Autodesk Inventor part; units mm, degrees
ref_plane "YZ Plane" through (0, 0, 0) normal (1, 0, 0) x (0, 1, 0)
ref_plane "XZ Plane" through (0, 0, 0) normal (0, 1, 0) x (-1, 0, 0)
ref_plane "XY Plane" through (0, 0, 0) normal (0, 0, 1) x (1, 0, 0)
sketch "Boceto1" plane through (0, 0, 0) normal (0, 1, 0) x (-1, 0, 0)
  line L0 (100, 100) -> (-100, 100)
  line L1 (-100, 100) -> (-100, -100)
  line L2 (-100, -100) -> (100, -100)
  line L3 (100, -100) -> (100, 100)
  line L4 (100, 100) -> (-100, -100) construction
  line L5 (-100, 100) -> (100, -100) construction
  point P0 (0, 0)
  dimension "d0" = 200
  dimension "d1" = 200
extrude "Extrusión1" add sketch "Boceto1" along normal blind 20
sketch "Boceto2" plane through (0, 20, 0) normal (0, 1, 0) x (1, 0, 0)
  circle A0 centre (-11.5239, -30.0616) radius 3
  circle A1 centre (11.4761, -30.0616) radius 3
  circle A2 centre (-11.5239, -60.0616) radius 3
  circle A3 centre (11.4761, -60.0616) radius 3
  line L0 (-0.0239, -45.0616) -> (-35.0239, -45.0616)
  line L1 (-35.0239, -45.0616) -> (-35.0239, -80.0616)
  line L2 (-0.0239, -45.0616) -> (34.9761, -45.0616)
  line L3 (-11.5239, -30.0616) -> (11.4761, -60.0616)
  line L4 (-11.5239, -60.0616) -> (11.4761, -30.0616)
  line L5 (34.9761, -20.0616) -> (-35.0239, -20.0616)
  line L6 (-35.0239, -20.0616) -> (-35.0239, -80.0616)
  line L7 (34.9761, -80.0616) -> (34.9761, -20.0616)
  line L8 (-105, -100.0616) -> (105, -100.0616)
  line L9 (-105.0239, -80.0616) -> (104.9761, -80.0616)
  line L10 (-35.0239, -80.0616) -> (34.9761, -80.0616)
  line L11 (105, -100.0616) -> (95.8154, -100.0616)
  line L12 (-105.0239, -80.0616) -> (104.9761, -80.0616)
  line L13 (105, -80.0616) -> (-105, -80.0616)
  line L14 (-105, -100.0616) -> (105, -100.0616)
  line L15 (105, -90.0616) -> (94.0798, -90.0616)
  line L16 (-105, -100.0616) -> (105, -100.0616)
  line L17 (-105, -80.0616) -> (105, -80.0616)
  line L18 (105, -80.0616) -> (105, -100.0616)
  line L19 (105, -100.0616) -> (-105, -100.0616)
  line L20 (-105, -100.0616) -> (-105, -80.0616)
  line L21 (-100, 100) -> (-100, -100)
  line L22 (-100, -100) -> (100.4077, -100)
  point P0 (0, 0)
  point P1 (0, -10.0616)
  point P2 (0, -90.0616)
  point P3 (-0.0478, -80.0616)
  dimension "d4" = 20
  dimension "d5" = 20
  dimension "d6" = 30
  dimension "d7" = 30
  dimension "d8" = 20
  dimension "d9" = 35
  dimension "d10" = 35
  dimension "d11" = 60
extrude "Extrusión2" cut sketch "Boceto2" against normal blind 10
sketch "Boceto3" plane through (0, 20, 0) normal (0, 1, 0) x (1, 0, 0)
  circle A0 centre (-11.5239, -30.0616) radius 3
  circle A1 centre (-11.5239, -30.0616) radius 3
  circle A2 centre (11.4761, -30.0616) radius 3
  circle A3 centre (11.4761, -30.0616) radius 3
  circle A4 centre (11.4761, -60.0616) radius 3
  circle A5 centre (11.4761, -60.0616) radius 3
  circle A6 centre (-11.5239, -60.0616) radius 3
  point P0 (0, 0)
extrude "Extrusión3" cut sketch "Boceto3" against normal blind 20
sketch "Boceto4" plane through (0, 20, 0) normal (0, 1, 0) x (1, 0, 0)
  circle A0 centre (-51.75, 78.25) radius 1.75
  line L0 (-50, 70) -> (-60, 70)
  line L1 (-60, 70) -> (-60, 80)
  line L2 (-60, 80) -> (-50, 80)
  line L3 (-50, 80) -> (-50, 70)
  line L4 (-50, 70) -> (-60, 80) construction
  line L5 (-60, 70) -> (-50, 80) construction
  line L6 (-105, 90) -> (-105, -90)
  circle A1 centre (-58.25, 71.75) radius 1.75
  line L7 (0, 90) -> (0, 77.3124)
  circle A2 centre (51.75, 78.25) radius 1.75
  line L8 (50, 70) -> (60, 70)
  line L9 (60, 70) -> (60, 80)
  line L10 (60, 80) -> (50, 80)
  line L11 (50, 80) -> (50, 70)
  line L12 (50, 70) -> (60, 80) construction
  line L13 (60, 70) -> (50, 80) construction
  circle A3 centre (58.25, 71.75) radius 1.75
  line L14 (100, 100) -> (-100, 100)
  line L15 (-100, 100) -> (-100, -80.0616)
  line L16 (100, -80.0616) -> (100, 100)
  point P0 (0, 0)
  point P1 (0, 0)
  point P2 (-60, 75)
  point P3 (60, 75)
  dimension "d16" = 3.5
  dimension "d18" = 1.75
  dimension "d19" = 1.75
  dimension "d20" = 1.75
  dimension "d21" = 1.75
  dimension "d22" = 10
  dimension "d23" = 10
  dimension "d25" = 20
  dimension "d26" = 40
  dimension "d27" = 40
hole "Agujero1" at (-58.25, 20, -71.75) at (-51.75, 20, -78.25) at (58.25, 20, -71.75) at (51.75, 20, -78.25) direction (0, -1, 0) diameter 3.5 end through all
sketch "Boceto5" plane through (0, 20, 0) normal (0, 1, 0) x (1, 0, 0)
  line L0 (0, 90) -> (0, 68.25)
  circle A0 centre (-51.75, 78.25) radius 1.75
  line L1 (-50, 78.25) -> (-50, 100)
  circle A1 centre (-58.25, 71.75) radius 1.75
  line L2 (-60, 71.75) -> (-60, 100)
  line L3 (-60, 100) -> (-70, 100)
  line L4 (-50, 100) -> (-40, 100)
  line L5 (-40, 100) -> (-40, 60)
  line L6 (-40, 60) -> (-70, 60)
  line L7 (-70, 60) -> (-70, 100)
  line L8 (-70, 100) -> (-40, 100)
  circle A2 centre (51.75, 78.25) radius 1.75
  line L9 (50, 78.25) -> (50, 100)
  circle A3 centre (58.25, 71.75) radius 1.75
  line L10 (60, 71.75) -> (60, 100)
  line L11 (60, 100) -> (70, 100)
  line L12 (50, 100) -> (40, 100)
  line L13 (40, 100) -> (40, 60)
  line L14 (40, 60) -> (70, 60)
  line L15 (70, 60) -> (70, 100)
  line L16 (70, 100) -> (40, 100)
  point P0 (0, 0)
  dimension "d38" = 10
  dimension "d39" = 10
  dimension "d40" = 40
extrude "Extrusión4" cut sketch "Boceto5" against normal blind 10
ref_plane "Plano de trabajo1" through (0, 0, -100) normal (-1, 0, 0) x (0, 0, 1)
ref_plane "Plano de trabajo2" through (100, 0, 0) normal (0, 0, -1) x (-1, 0, 0)
sketch "Boceto7" plane through (0, 0, 0) normal (0, -1, 0) x (1, 0, 0)
  circle A0 centre (10, -10) radius 1.75
  line L0 (6.803, 0) -> (14.6069, 0)
  line L1 (0, 0) -> (0, -4.8284)
  line L2 (0, 0) -> (20.0354, 0)
  circle A1 centre (10, 10) radius 1.75
  line L3 (0, 0) -> (0, 4.8284)
  circle A2 centre (-10, -10) radius 1.75
  circle A3 centre (-10, 10) radius 1.75
  dimension "d52" = 3.5
  dimension "d54" = 10
  dimension "d55" = 10
hole "Agujero2" at (10, 0, -10) at (10, 0, 10) at (-10, 0, 10) at (-10, 0, -10) direction (0, 1, 0) diameter 3.5 end through all
sketch "Boceto8" plane through (0, 0, 0) normal (0, -1, 0) x (1, 0, 0)
  line L0 (-15, 15) -> (15, 15)
  line L1 (15, 15) -> (15, -15)
  line L2 (15, -15) -> (-15, -15)
  line L3 (-15, -15) -> (-15, 15)
  line L4 (-15, 15) -> (15, -15) construction
  line L5 (15, 15) -> (-15, -15) construction
  point P0 (0, 0)
  dimension "d63" = 30
  dimension "d64" = 30
extrude "Extrusión5" cut sketch "Boceto8" against normal blind 10
sketch "Boceto9" plane through (0, 0, 0) normal (0, -1, 0) x (1, 0, 0)
  circle A0 centre (85, -10) radius 1.75
  line L0 (100, 100) -> (100, -100)
  line L1 (140, 0) -> (-140, 0)
  circle A1 centre (85, 10) radius 1.75
  line L2 (0, 0) -> (0, 9.4908)
  circle A2 centre (-85, -10) radius 1.75
  circle A3 centre (-85, 10) radius 1.75
  line L3 (0, 0) -> (6.3157, 6.3157)
  line L4 (0, 0) -> (8.9318, 0) construction
  circle A4 centre (10, 85) radius 1.75
  circle A5 centre (-10, -85) radius 1.75
  line L5 (0, 0) -> (5.9531, -5.9531)
  line L6 (0, 0) -> (8.419, 0) construction
  circle A6 centre (10, -85) radius 1.75
  circle A7 centre (-10, 85) radius 1.75
  dimension "d67" = 3.5
  dimension "d68" = 15
  dimension "d69" = 10
  dimension "d70" = 45
  dimension "d71" = 45
hole "Agujero3" at (-10, 0, 85) at (10, 0, 85) at (85, 0, 10) at (85, 0, -10) at (-85, 0, 10) at (-85, 0, -10) at (-10, 0, -85) at (10, 0, -85) direction (0, 1, 0) diameter 3.5 end through all
split "Dividir3" plane through (100, 0, 0) removes the side toward (0, 0, -1)
split "Dividir4" plane through (0, 0, -100) removes the side toward (1, 0, 0)
properties part number "base_front_3"
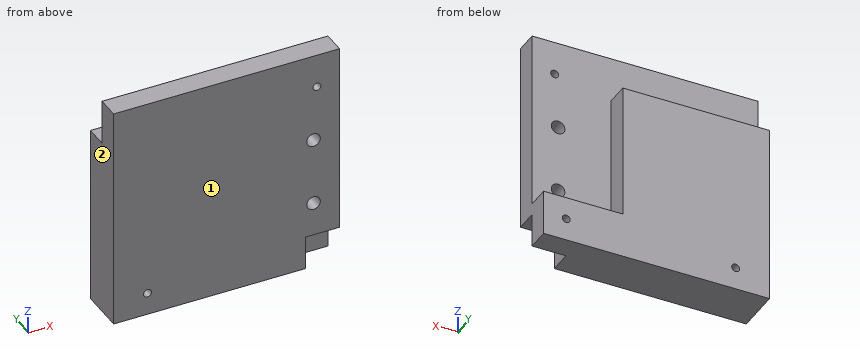
CAD build for the part. Positions are in the model's coordinates, mm. Face numbers are marked on the shaded views. Round coordinates to 2 decimals unless told otherwise and drop trailing zeros. Write each loop counter-clockwise with the first axis right and the second up, starting at its lowest first coordinate (ties: lowest second). Pieces come first, ordered by that corner, then holes. Notation, with made-up numbers: (-13, -26) -> (12, -26) arc R29 ccw to (12, 8) -> close; hole circle Ø5 at (39.25, -9). An arc over 180 degrees is marked (long way). Answer in a Markdown table with one row per item. Add a question column.
Item 1: Drop flat-ended pins along their axis: pin 1 Ø8 at (x, y) = (-10.5, 13.5) entering from +Z; pin 2 Ø4.5 at (x, z) = (-4, 10) entering from -Y; pin 3 Ø3 at (y, z) = (4, 7) entering from +X; pin 4 Ø5.5 at (x, z) = (-11.52, 60.06) entering from +Y. Give the stop position or say it passes through.
Item 2: Saw through at D-D, the plane x = -10. Write the cut outline in (y, z), then the cut area to 3 significant figures.
Item 3: Drill centre lines: line 1 (X direction, y = 12.5, z = 10); line 2 (Z direction, x = -61.5, y = 16); line 3 (X direction, y = 12.75, z = 73.5). Where is each one in solid material? Low to high. Write a range as from..to.
Item 4: Saw through at A-A, the plane x = -85. Write the cut outline in (y, z).
Item 5: Saw through at C-C, the plane z = 85. Write the cut outline in (x, y), then the cut area to 3 significant figures.
Item 6: Saw through at B-B, the plane z = 10. Write the cut outline in (x, y).
Item 7: Mould opens along X. For the marked faces 1 and 2 say: pulls with the +X half, pulls with the -X half, needs draft (parallel to the pull), parting line crosses it, or undercut.
Findings below:
| question | item | result |
|---|---|---|
| 1 | pin 1 | stops at z = 100 |
| 1 | pin 2 | stops at y = 10 |
| 1 | pin 3 | stops at x = -15 |
| 1 | pin 4 | passes through |
| 2 | outline | (0, 15) -> (10, 15) -> (10, 11.75) -> (20, 11.75) -> (20, 20.06) -> (10, 20.06) -> (10, 27.48) -> (0, 27.48) -> close; (0, 32.65) -> (10, 32.65) -> (10, 57.48) -> (0, 57.48) -> close; (0, 62.65) -> (10, 62.65) -> (10, 83.25) -> (0, 83.25) -> close; (0, 86.75) -> (10, 86.75) -> (10, 100) -> (0, 100) -> close; (10, 0) -> (20, 0) -> (20, 8.25) -> (10, 8.25) -> close |
| 2 | area | 877 mm^2 |
| 3 | line 1 | x = -100..-86.75, -83.25..-11.75, -8.25..0 |
| 3 | line 2 | z = 0..80.06 |
| 3 | line 3 | x = -100..-35.02 |
| 4 | outline | (0, 0) -> (20, 0) -> (20, 8.25) -> (0, 8.25) -> close; (0, 11.75) -> (20, 11.75) -> (20, 80.06) -> (10, 80.06) -> (10, 100) -> (0, 100) -> close |
| 5 | outline | (-100, 0) -> (-11.75, 0) -> (-11.75, 10) -> (-100, 10) -> close; (-8.25, 0) -> (0, 0) -> (0, 10) -> (-8.25, 10) -> close |
| 5 | area | 965 mm^2 |
| 6 | outline | (-100, 0) -> (-86.75, 0) -> (-86.75, 20) -> (-100, 20) -> close; (-83.25, 0) -> (-15, 0) -> (-15, 10) -> (-11.75, 10) -> (-11.75, 20) -> (-83.25, 20) -> close; (-8.25, 10) -> (0, 10) -> (0, 20) -> (-8.25, 20) -> close |
| 7 | face 1 | needs draft |
| 7 | face 2 | pulls with the -X half |
